```python
from build123d import *

# Parameters (mm, degrees)
SKETCH1_W                = 46
SKETCH1_H                = 20
BOSS_EXTRUDE1_DEPTH      = 10
BOSS_EXTRUDE2_DEPTH      = 5
BOSS_EXTRUDE2_DEPTH_BACK = 10
SKETCH3_W                = 38
SKETCH3_H                = 20
CUT_EXTRUDE1_DEPTH       = 7
CHAMFER1_START           = -38.660254038
CHAMFER1_DEPTH           = 48.660254038


with BuildPart() as part:
    # Sketch1 → Boss-Extrude1 (new body)
    # profile 1 of 3: a face of its own
    with BuildSketch(Plane.XY):
        Rectangle(SKETCH1_W, SKETCH1_H)
        with BuildLine():
            Line((-13.45, 7), (-13.45, 0))
            Line((-13.45, 0), (-13.45, -7))
            ThreePointArc((-13.45, -7), (-15, -8.55), (-16.55, -7))
            Line((-16.55, -7), (-16.55, -2.8e-08))
            Line((-16.55, -2.8e-08), (-16.55, 7))
            ThreePointArc((-16.55, 7), (-15, 8.55), (-13.45, 7))
        make_face(mode=Mode.SUBTRACT)
        with BuildLine():
            Line((13.45, -7), (13.45, -7e-09))
            Line((13.45, -7e-09), (13.45, 7))
            ThreePointArc((13.45, 7), (15, 8.55), (16.55, 7))
            Line((16.55, 7), (16.55, 0))
            Line((16.55, 0), (16.55, -7))
            ThreePointArc((16.55, -7), (15, -8.55), (13.45, -7))
        make_face(mode=Mode.SUBTRACT)
    # profile 2 of 3: a face of its own
    with BuildSketch(Plane.XY):
        Polygon((-23, -30), (-23, -10), (-23, 10), (-27, 10), (-27, -30), align=None)
    # profile 3 of 3: a face of its own
    with BuildSketch(Plane.XY):
        Polygon((23, 10), (23, -10), (23, -30), (27, -30), (27, 10), align=None)
    extrude(amount=BOSS_EXTRUDE1_DEPTH)

    # Sketch2 → Boss-Extrude2 (add, two sides: drawn at the far end of the back side and taken through both)
    with BuildSketch(Plane(origin=(0, 0, 0), x_dir=(-1, 0, 0), z_dir=(0, 0, -1)).offset(-BOSS_EXTRUDE2_DEPTH_BACK)):
        Polygon((-23, -30), (-38, -38.660254038), (-38, -30), align=None)
        Polygon((23, -30), (38, -38.660254038), (38, -30), align=None)
    extrude(amount=BOSS_EXTRUDE2_DEPTH + BOSS_EXTRUDE2_DEPTH_BACK)

    # Sketch3 → Cut-Extrude1 (cut)
    with BuildSketch(Plane(origin=(0, 0, 0), x_dir=(-1, 0, 0), z_dir=(0, 0, -1))):
        Rectangle(SKETCH3_W, SKETCH3_H)
    extrude(amount=-CUT_EXTRUDE1_DEPTH, mode=Mode.SUBTRACT)

    # Chamfer1: read off the stored shape, not the designer's step
    # Chamfer1 outline → Chamfer1 (cut)
    with BuildSketch(Plane(origin=(0, 0, 0), x_dir=(1, 0, 0), z_dir=(0, 1, 0)).offset(CHAMFER1_START)):
        Polygon((-23, 5), (-31, 5), (-19, -7), (-19, 0), (-23, 0), align=None)
        Polygon((31, 5), (23, 5), (23, 0), (19, 0), (19, -7), align=None)
    extrude(amount=CHAMFER1_DEPTH, mode=Mode.SUBTRACT)


solid = part.part
```
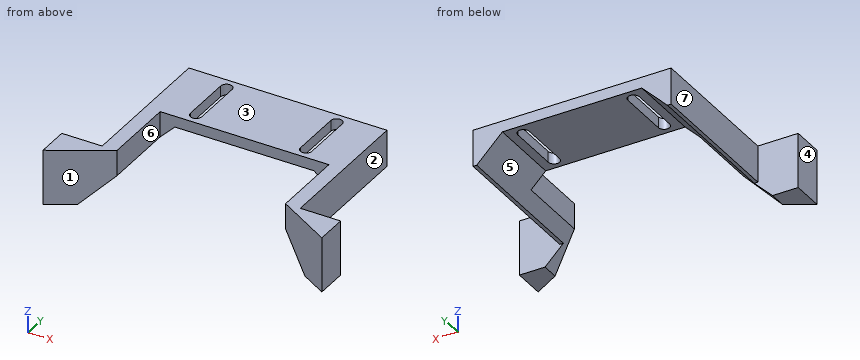
CAD build for the part. Positions are in the model's coordinates, mm. Face numbers are marked on the shaded views. A direction names the side the tool comes from. Round coordinates to 2 decimals unless told otherwise and drop trailing zeros. Order: outer loops, then holes, each group sorted by start corner. A loop starts at its lowest first (then second) coordinate and runs counter-clockwise, first axis right, second up. Notation, with made-up numbers: (66.25, 0) -> (111.25, 0) arc R28 cw to (111.25, 27) -> close; hole circle Ø6 at (29, 32.25). An arc over 180 degrees is marked (long way). One line per question, with ' | ' between items.
Q1. Drop flat-ended pins along their axis: pin 1 (5.5 mm diameter, centred on y = -19, z = 5, fed in from +X); pin 2 (0.8 mm diameter, centred on x = -26.5, y = -10.5, fed in from -Z); pin 3 (3.5 mm diameter, centred on x = 3, z = 6, fed in from -Y). Give the stop position or say it passes through.
Completed:
pin 1: stops at x = 27 | pin 2: stops at z = 0 | pin 3: stops at y = -10
Q2. Slice it at D-D (y = -24.5). Write the cut outline in (x, z).
Completed:
outline: (-27, 0) -> (-26, 0) -> (-23, 3) -> (-23, 10) -> (-27, 10) -> close; (23, 3) -> (26, 0) -> (27, 0) -> (27, 10) -> (23, 10) -> close
Q3. Slice it at A-A (x = -15). Write the cut outline in (y, z), then the cut area to 3 significant figures.
Completed:
outline: (-10, 7) -> (-8.55, 7) -> (-8.55, 10) -> (-10, 10) -> close; (8.55, 7) -> (10, 7) -> (10, 10) -> (8.55, 10) -> close | area: 8.70 mm^2
Q4. Which spindle directions (+Z, -Z, +X, -X, +Y, -Y) get a long thin tool onto all of the face, cutting with end or side? Do the marked faces 4, 5, 6 and 7. Say none if no direction does.
Completed:
face 4: +Z, -Z, -X, +Y, -Y | face 5: -Z, +Y, -Y | face 6: +Z, -Z, -Y | face 7: +Z, -Z, -X, +Y
Q5. Slice it at B-B (y = -1). Write the cut outline in (x, z).
Completed:
outline: (-27, 0) -> (-26, 0) -> (-19, 7) -> (-16.55, 7) -> (-16.55, 10) -> (-27, 10) -> close; (-13.45, 7) -> (13.45, 7) -> (13.45, 10) -> (-13.45, 10) -> close; (16.55, 7) -> (19, 7) -> (26, 0) -> (27, 0) -> (27, 10) -> (16.55, 10) -> close
Q6. Probe probe 1 along X at (y, z) = (-15, 5.5); probe 2 along Z at (x, y) = (3, 1); probe 3 along X at (y, z) = (2, 0.75). List the from-to ranges inside material, lowest first.
Completed:
probe 1: x = -27 to -23, 23 to 27 | probe 2: z = 7 to 10 | probe 3: x = -27 to -25.25, 25.25 to 27
Q7. Slice it at C-C (z = -4). Write the cut outline in (x, y).
Completed:
outline: (-38, -38.66) -> (-30, -34.04) -> (-30, -30) -> (-38, -30) -> close; (30, -34.04) -> (38, -38.66) -> (38, -30) -> (30, -30) -> close
Q8. Two-plate mould, pull along X, no slides. Class the marked faces 1, 2 and 3: released by +X, released by -X, zero draft, split by the parting line, or undercut.
Completed:
face 1: undercut | face 2: released by +X | face 3: zero draft
